```python
from build123d import *

# Parameters (mm, degrees)
CROQUIS7_R              = 3
CROQUIS7_R_2            = 1.5
SALIENTE_EXTRUIR4_DEPTH = 4
CROQUIS9_R              = 1.5
CROQUIS9_R_2            = 1.25
SALIENTE_EXTRUIR5_DEPTH = 4
CROQUIS2_R              = 3.020046414
CROQUIS2_R_2            = 1.5
SALIENTE_EXTRUIR2_DEPTH = 4
CHAFL_N1_SIZE           = 0.5


with BuildPart() as part:
    # Croquis7 → Saliente-Extruir4 (new body)
    with BuildSketch(Plane.XY):
        Circle(CROQUIS7_R)
        Circle(CROQUIS7_R_2, mode=Mode.SUBTRACT)
    extrude(amount=-SALIENTE_EXTRUIR4_DEPTH)

    # Croquis9 → Saliente-Extruir5 (add)
    with BuildSketch(Plane.XY):
        with BuildLine():
            Line((0.210526316, 3.994455992), (19.157894737, 2.995841994))
            ThreePointArc((19.157894737, 2.995841994), (22, 0), (19.157894737, -2.995841994))
            Line((19.157894737, -2.995841994), (0.210526316, -3.994455992))
            ThreePointArc((0.210526316, -3.994455992), (-4, 0), (0.210526316, 3.994455992))
        make_face()
        Circle(CROQUIS9_R, mode=Mode.SUBTRACT)
        with Locations((19, 0)):
            Circle(CROQUIS9_R_2, mode=Mode.SUBTRACT)
    extrude(amount=-SALIENTE_EXTRUIR5_DEPTH)

    # Croquis2 → Saliente-Extruir2 (add, through all)
    with BuildSketch(Plane.XY.offset(-4)):
        with BuildLine():
            Line((-3.171102714, 20.998669186), (3.771863049, 1.331558915))
            ThreePointArc((3.771863049, 1.331558915), (1.149391542, -3.831305141), (-3.881954792, -0.964586438))
            Line((-3.881954792, -0.964586438), (-8.911466094, 19.276560172))
            ThreePointArc((-8.911466094, 19.276560172), (-6.862043657, 22.873478856), (-3.171102714, 20.998669186))
        make_face()
        Circle(CROQUIS2_R, mode=Mode.SUBTRACT)
        with Locations((-6, 20)):
            Circle(CROQUIS2_R_2, mode=Mode.SUBTRACT)
    extrude(amount=SALIENTE_EXTRUIR2_DEPTH)

    # Chaflán1
    chafl_n1_edges = [part.edges().sort_by_distance(p)[0] for p in [
        (11.01969335, 3.424762868, -4),
        (22, 0, -4),
        (9.684210526, -3.495148993, -4),
        (9.684210526, -3.495148993, 0),
        (22, 0, 0),
        (11.01969335, 3.424762868, 0),
        (-2.380099608, -3.214829056, 0),
        (-2.380099608, -3.214829056, -4),
        (-6.396710443, 9.155986867, 0),
        (-0.144805375, 12.426176464, 0),
        (-6.862043657, 22.873478856, 0),
        (-6.862043657, 22.873478856, -4),
        (-6.396710443, 9.155986867, -4),
        (-0.144805375, 12.426176464, -4),
    ]]
    chamfer(chafl_n1_edges, length=CHAFL_N1_SIZE)


solid = part.part
```
Build history of the part. All positions in model axes, mm. Round coordinates to 2 decimals unless told otherwise and drop trailing zeros. Loops run counter-clockwise (first coordinate to the right, second up) from the corner with the lowest first, then second, coordinate; pieces in that order, holes last.
Item 1: Two-plate mould, pull along Y, no slides. Class faces 1 (the face through (10.72, 3.19, -3.75)), 2 (the face through (-1.5, 0.07, -1.97)), 3 (the face through (1, 5, -4)): released by +Y, released by -Y, zero draft, split by the parting line, or undercut.
Item 2: Drill centre lines: line 1 along Y through (x, z) = (19, -0.9); line 2 along X through (y, z) = (1, -0.3); line 3 along Y through (x, z) = (20, -0.95). Where is each one in solid material? Low to high.
Item 3: Saw through at A-A (z = -2.3). List the corners of the cut face in (x, y), then the cut area to 3 significant figures.
Item 4: Pin check, flat tips, straight feed: P1, Ø5, axis at x = 0, y = 0, coming from the -Z side; P2, Ø1, axis at x = 4, z = -2.5, coming from the -Y side; P3, Ø2.5, axis at x = -6, y = 20, coming from the -Z side; P4, Ø1, axis at y = 8, z = -1.5, coming from the -X side. Stop position of each tip, or through.
Item 5: Saw through at C-C (y = 0). List the corners of the cut face in (x, z), then the cut area to 3 significant figures.
Item 6: Saw through at D-D (x = -6). List the corners of the cut face in (y, z).
Item 7: Saw through at B-B (y = 20). List the corners of the cut face in (x, z).
Worked answers:
1. face 1: released by +Y
1. face 2: undercut
1. face 3: zero draft
2. line 1: y = -3 to -1.25, 1.25 to 3
2. line 2: x = -4.16 to -1.12, 1.12 to 18.25, 19.75 to 21.62
2. line 3: y = -2.83 to -0.75, 0.75 to 2.83
3. outline: (-8.91, 19.28) - (-3.88, -0.96) arc R4 ccw to (0.21, -3.99) - (19.16, -3) arc R3 ccw to (19.16, 3) - (2.88, 3.85) - (-3.17, 21) arc R3 ccw to start; hole circle Ø3 at (-6, 20); hole circle Ø3 at (0, 0); hole circle Ø2.5 at (19, 0)
3. area: 287 mm2
4. P1: stops at z = -4
4. P2: stops at y = -3.82
4. P3: passes through
4. P4: stops at x = -6.23
5. outline: (-4.12, -3.5) - (-3.61, -4) - (-1.5, -4) - (-1.5, 0) - (-3.61, 0) - (-4.12, -0.5) - close; (1.5, -4) - (17.75, -4) - (17.75, 0) - (1.5, 0) - close; (20.25, -4) - (21.5, -4) - (22, -3.5) - (22, -0.5) - (21.5, 0) - (20.25, 0) - close
5. area: 82.0 mm2
6. outline: (7.56, -3.5) - (9.63, -4) - (18.5, -4) - (18.5, 0) - (9.63, 0) - (7.56, -0.5) - close; (21.5, -4) - (22.5, -4) - (23, -3.5) - (23, -0.5) - (22.5, 0) - (21.5, 0) - close
7. outline: (-9, -3.5) - (-8.5, -4) - (-7.5, -4) - (-7.5, 0) - (-8.5, 0) - (-9, -0.5) - close; (-4.5, -4) - (-3.35, -4) - (-2.82, -3.5) - (-2.82, -0.5) - (-3.35, 0) - (-4.5, 0) - close
